Part print with two shaded views. Sizes in mm from the minimum x, y, z corner. A direction names the side the tool comes from. Coordinates: 2 decimals unless noted, no trailing zeros. Loops run counter-clockwise (first coordinate to the right, second up) from the corner with the lowest first, then second, coordinate; pieces in that order, holes last. Notation, with made-up numbers: (-39.75, -24.75) -> (12.25, -24.75) arc R32 cw to (12.25, 7.25) -> close; hole circle Ø1 at (66, 15). An arc over 180 degrees is marked (long way). Return JSON: item names as keys, results as strings. Group by question number.
(1) Tool access for the marked faces 1, 2, 3, 4 and 5: list every direction of +Z, -Z, +X, -X, +Y, -Y with a clear straight run to the whole face (end or side of a thin tool).
(2) Saw through at A-A on y = 32.5. Write the cut outline in (x, z), then the cut area to 3 significant figures.
(3) Saw through at B-B on z = 26.5. Write the cut outline in (x, y) (1 decimal).
(4) Probe L1, parallel to X at y = 47, z = 5.5; L2, parallel to Z at x = 115.5, y = 36 (1 decimal); L3, parallel to Z at x = 64.5, y = 25. List the from-to ranges inside material, lowest first.
(5) Flat gauge pins, fed straight in: pin 1 Ø3 at (x, y) = (88, 43.5) entering from +Z; pin 2 Ø12 at (x, z) = (90, 5.5) entering from +Y; pin 3 Ø1.5 at (x, z) = (94, 35.5) entering from -Y. Where does each tip first touch, or does it go through?
(6) Saw through at C-C on x = 87. Write the cut outline in (y, z), then the cut area to 3 significant figures.
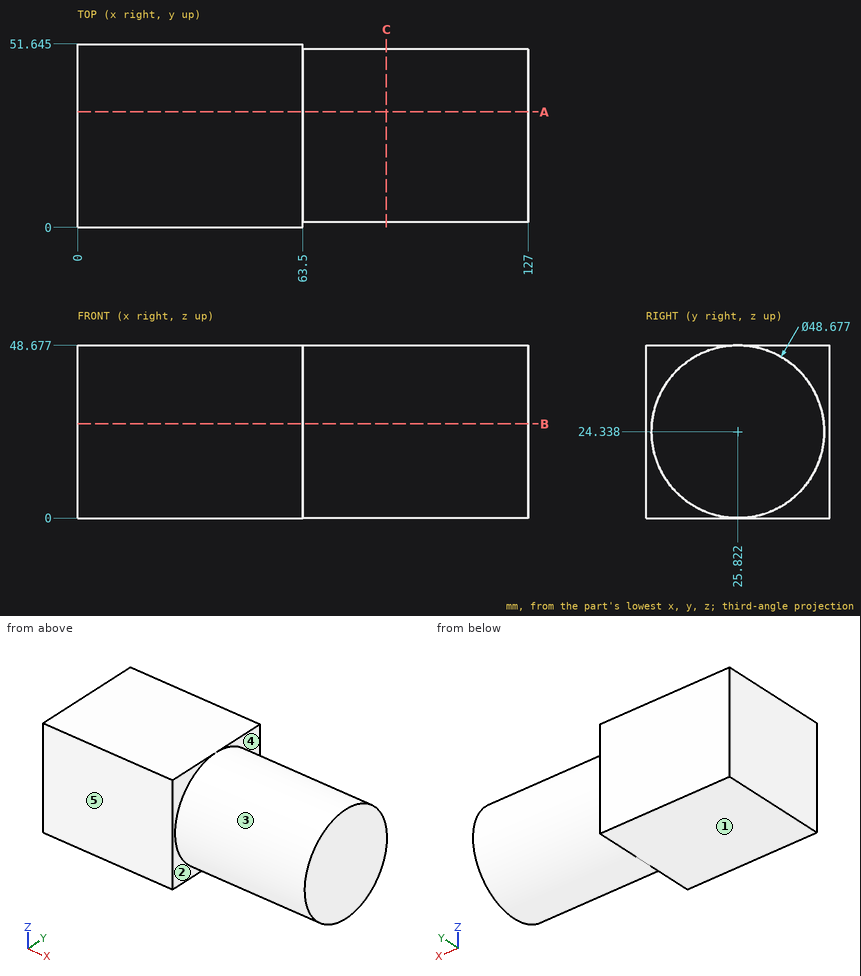
Geometry results:
{
 "1": {"face 1": "-Z, +X, -X, +Y, -Y", "face 2": "+X, -Y", "face 3": "+X", "face 4": "+X, +Y", "face 5": "+Z, -Z, +X, -X, -Y"},
 "2": {"outline": "(0, 0) -> (63.5, 0) -> (63.5, 0.93) -> (127, 0.93) -> (127, 47.74) -> (63.5, 47.74) -> (63.5, 48.68) -> (0, 48.68) -> close", "area": "6,060 mm²"},
 "3": {"outline": "(0, 0) -> (63.5, 0) -> (63.5, 1.6) -> (127, 1.6) -> (127, 50.1) -> (63.5, 50.1) -> (63.5, 51.6) -> (0, 51.6) -> close"},
 "4": {"L1": "0 to 63.5", "L2": "2.2 to 46.4", "L3": "0.01 to 48.66"},
 "5": {"pin 1": "z = 42.52", "pin 2": "y = 46.5", "pin 3": "y = 3.82"},
 "6": {"outline": "circle Ø48.68 at (25.82, 24.34)", "area": "1,860 mm²"}
}
